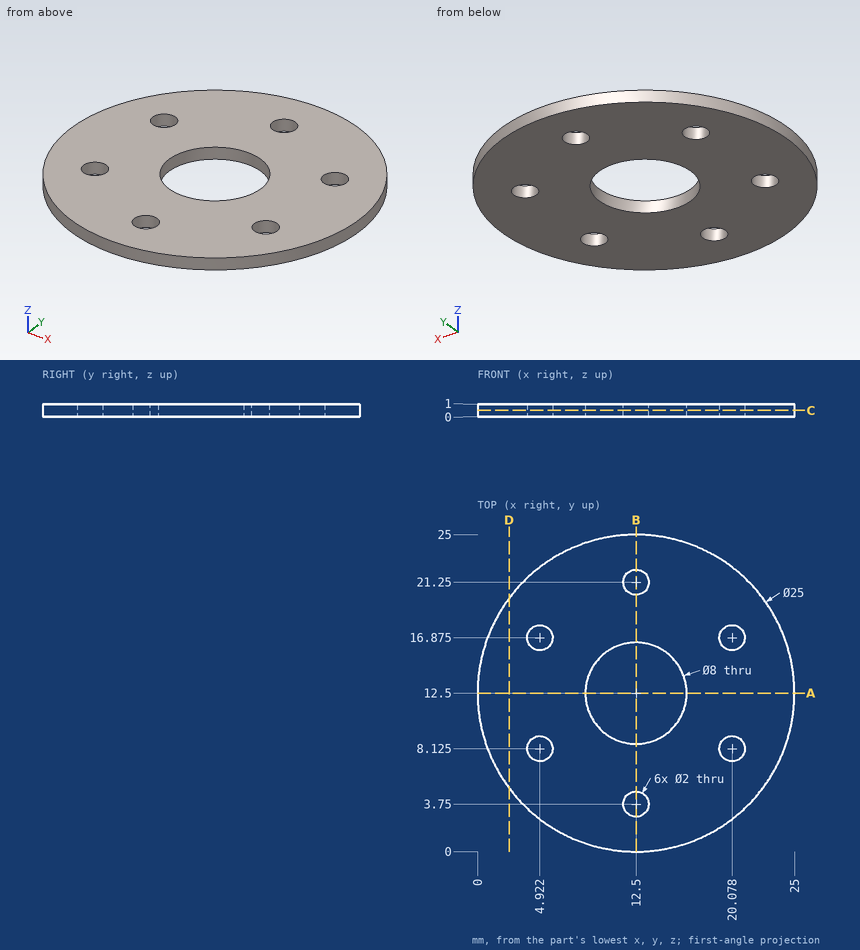
Input: dimensioned drawing with shaded views. Units: mm. Origin: part minimum x, y, z. Give positions to 0.01 mm unless a question says otherwise; leave off trailing zeros. Order: outer loops, then holes, each group sorted by start corner. A loop starts at its lowest first (then second) coordinate and runs counter-clockwise, first axis right, second up. Notation, with made-up numbers: (7.5, -14.5) -> (44.5, -14.5) arc R32 cw to (44.5, 11.5) -> close; hole circle Ø5 at (46.5, 8). An arc over 180 degrees is marked (long way). Use a Markdown table: item, result.
1) Section query D-D, the plane x = 2.5. Return the cut outline in (y, z), then the cut area to 3 significant figures.
Answer list:
| item | result |
|---|---|
| outline | (5, 0) -> (20, 0) -> (20, 1) -> (5, 1) -> close |
| area | 15.0 mm² |
2) Section query A-A, the plane y = 12.5. Return the cut outline in (x, z), then the cut area to 3 significant figures.
Answer list:
| item | result |
|---|---|
| outline | (0, 0) -> (8.5, 0) -> (8.5, 1) -> (0, 1) -> close; (16.5, 0) -> (25, 0) -> (25, 1) -> (16.5, 1) -> close |
| area | 17.0 mm² |
3) Contact query for flat-ended pins moving along their axis: P1, Ø2.5, axis at x = 20.08, y = 8.12, coming from the +Z side; P2, Ø1.6, axis at x = 4.92, y = 16.88, coming from the +Z side. Output: stop coordinate, or through.
Answer list:
| item | result |
|---|---|
| P1 | z = 1 |
| P2 | through |
4) Section query B-B, the plane x = 12.5. Return the cut outline in (y, z).
Answer list:
| item | result |
|---|---|
| outline | (0, 0) -> (2.75, 0) -> (2.75, 1) -> (0, 1) -> close; (4.75, 0) -> (8.5, 0) -> (8.5, 1) -> (4.75, 1) -> close; (16.5, 0) -> (20.25, 0) -> (20.25, 1) -> (16.5, 1) -> close; (22.25, 0) -> (25, 0) -> (25, 1) -> (22.25, 1) -> close |
5) Section query C-C, the plane z = 0.5. Count the separate pieces of the cut face and the enclosed holes in it, then the cut area to 3 significant figures.
Answer list:
| item | result |
|---|---|
| separate pieces | 1 |
| enclosed holes | 7 |
| area | 422 mm² |
6) Ray query, line 1 along Y through (x, z) = (12.5, 0.5); line 2 along Y through (x, z) = (4.5, 0.1) (1 decimal); line 3 along Y through (x, z) = (12, 0.1) (1 decimal). Return the intervals inside material, ascending. Write a range as [from, to].
Answer list:
| item | result |
|---|---|
| line 1 | [0, 2.75], [4.75, 8.5], [16.5, 20.25], [22.25, 25] |
| line 2 | [2.9, 7.2], [9, 16], [17.8, 22.1] |
| line 3 | [0, 2.9], [4.6, 8.5], [16.5, 20.4], [22.1, 25] |
